Design review of the part shown in the three views and the two pictorial views. Dimensions are in mm from the part's minimum x, y and z. A direction names the side the tool comes from. Round coordinates to 2 decimals unless told otherwise and drop trailing zeros. Order: outer loops, then holes, each group sorted by start corner. A loop starts at its lowest first (then second) coordinate and runs counter-clockwise, first axis right, second up.
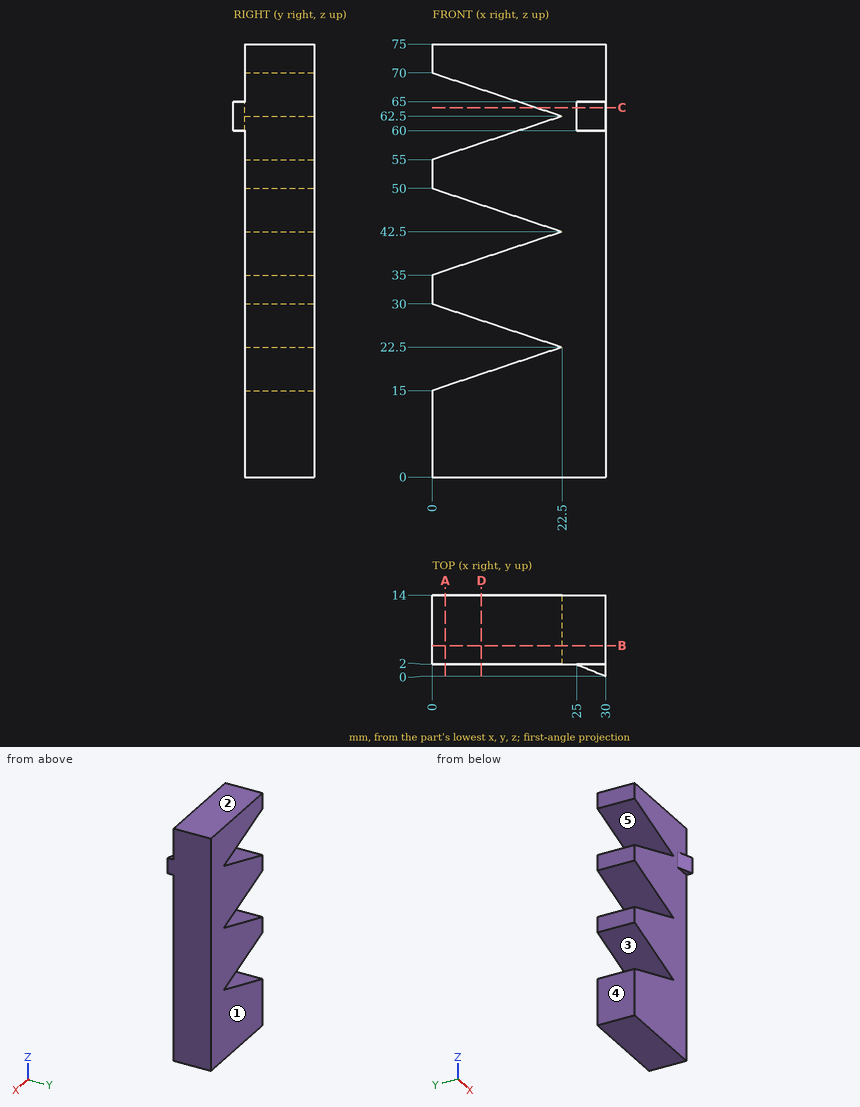
(1) Draft analysis for pull direction Z (two halves, no side actions). For the marked faces 1, 2 and 3, state which applies: pulls with the +Z half, pulls with the -Z half, needs draft (parallel to the pull), parting line crosses it, or undercut.
Data:
face 1: needs draft
face 2: pulls with the +Z half
face 3: undercut
(2) For the marked faces 4 and 5, list the 3-axis set-ups (+Z, -Z, +X, -X, +Y, -Y) from which the entire face can be reached by the end or side of a thin tool; tool diameter is ignored.
Data:
face 4: +Z, -Z, -X, +Y, -Y
face 5: -X, +Y, -Y
(3) To check wall thickness, follow probe 1 along Z at (x, y) = (18.25, 7.5); probe 2 along Z at (x, y) = (2, 10); probe 3 along Y at (x, z) = (24, 3). State the ranges of each line that lie inside material, in increasing order.
Data:
probe 1: z = 0 to 21.08, 23.92 to 41.08, 43.92 to 61.08, 63.92 to 75
probe 2: z = 0 to 15.67, 29.33 to 35.67, 49.33 to 55.67, 69.33 to 75
probe 3: y = 2 to 14
(4) Consider section C-C (z = 64). Write out the cut boundary in (x, y), and give its area (3 significant figures).
Data:
outline: (18, 2) - (25, 2) - (30, 0) - (30, 14) - (18, 14) - close
area: 149 mm2
(5) Consider section B-B (y = 5.25). Write out the cut boundary in (x, z), and give its area (3 significant figures).
Data:
outline: (0, 0) - (30, 0) - (30, 75) - (0, 75) - (0, 70) - (22.5, 62.5) - (0, 55) - (0, 50) - (22.5, 42.5) - (0, 35) - (0, 30) - (22.5, 22.5) - (0, 15) - close
area: 1,740 mm2
(6) Consider section A-A (x = 2.25). Write out the cut boundary in (y, z), and give its area (3 significant figures).
Data:
outline: (2, 0) - (14, 0) - (14, 15.75) - (2, 15.75) - close; (2, 29.25) - (14, 29.25) - (14, 35.75) - (2, 35.75) - close; (2, 49.25) - (14, 49.25) - (14, 55.75) - (2, 55.75) - close; (2, 69.25) - (14, 69.25) - (14, 75) - (2, 75) - close
area: 414 mm2
(7) Consider section D-D (x = 8.5). Write out the cut boundary in (y, z).
Data:
outline: (2, 0) - (14, 0) - (14, 17.83) - (2, 17.83) - close; (2, 27.17) - (14, 27.17) - (14, 37.83) - (2, 37.83) - close; (2, 47.17) - (14, 47.17) - (14, 57.83) - (2, 57.83) - close; (2, 67.17) - (14, 67.17) - (14, 75) - (2, 75) - close
(8) Insertion check: pin 1 (2 mm diameter, centred on x = 13, z = 21.5, fed in from -Y) (3 decimals); pin 2 (0.6 mm diameter, centred on x = 27, y = 1, fed in from +Z). Each pin has a flat end and moves straight along its axis. Give the tip position at first contact, or say it passes through.
Data:
pin 1: passes through
pin 2: stops at z = 65
